Geometry: final body of the model. Coordinates: model frame, mm. Coordinates: 2 decimals unless noted, no trailing zeros. Write each loop counter-clockwise with the first axis right and the second up, starting at its lowest first coordinate (ties: lowest second). Pieces come first, ordered by that corner, then holes.
Autodesk Fusion 360 part; units mm, degrees
sketch "Esquisse1" plane through (0, 0, 0) normal (0, 0, 1) x (1, 0, 0)
  line L0 (74.9967, -34.0812) -> (-36.2033, -34.0812)
  circle A0 centre (59.0467, 6.2188) radius 15
  line L1 (76.9967, 28.1188) -> (76.9967, -32.0812)
  line L2 (-38.2033, -32.0812) -> (-38.2033, 28.1188)
  line L3 (74.8967, -31.9812) -> (-36.1033, -31.9812)
  line L4 (-36.2033, 30.1188) -> (74.9967, 30.1188)
  line L5 (-36.1033, 28.0188) -> (74.8967, 28.0188)
  line L6 (-36.1033, -31.9812) -> (-36.1033, 28.0188)
  circle A1 centre (8.0467, 6.2188) radius 15
  line L7 (74.8967, 28.0188) -> (74.8967, -31.9812)
  arc A2 (74.9967, -34.0812) -> (76.9967, -32.0812) centre (74.9967, -32.0812) ccw
  arc A3 (76.9967, 28.1188) -> (74.9967, 30.1188) centre (74.9967, 28.1188) ccw
  arc A4 (-36.2033, 30.1188) -> (-38.2033, 28.1188) centre (-36.2033, 28.1188) ccw
  arc A5 (-38.2033, -32.0812) -> (-36.2033, -34.0812) centre (-36.2033, -32.0812) ccw
  circle A6 centre (-19.1033, 10.5188) radius 6.5
  point P0 (-37.2797, 0.2421)
  dimension "d25" = 115.2
  dimension "d26" = 64.2
  dimension "d38" = 30
  dimension "d41" = 46.25
  dimension "d42" = 111
  dimension "d43" = 60
  dimension "d44" = 2.1
  dimension "d45" = 2.1
  dimension "d47" = 30
  dimension "d48" = 51
  dimension "d21" = 2
  dimension "d22" = 2
  dimension "d23" = 2
  dimension "d24" = 2
  dimension "d28" = 13
  dimension "d29" = 42.5
  dimension "d30" = 17
  dimension "d34" = 38.2
  dimension "d35" = 38.2
extrude "Extrusion1" add sketch "Esquisse1" along normal blind 1 contours L0 L1 L2 L4 A2 A3 A4 A5 | L3 L5 L6 L7
Item 1: Section B-B, the plane y = -2.5. Output: boundary loops of the cut face in (x, z), plus the area to 3 significant figures.
Derived:
outline: (-38.2, 0) - (-4.16, 0) - (-4.16, 1) - (-38.2, 1) - close; (20.25, 0) - (46.84, 0) - (46.84, 1) - (20.25, 1) - close; (71.25, 0) - (77, 0) - (77, 1) - (71.25, 1) - close
area: 66.4 mm2
Item 2: Pin query (flat end, axial travel): pin 1 (1.5 mm diameter, centred on x = 36, y = -22.5, fed in from -Z); pin 2 (8 mm diameter, centred on x = -19.1, y = 10.52, fed in from -Z). Return the tip coordinate at first contact, or that it passes through.
Derived:
pin 1: stops at z = 0
pin 2: passes through
Item 3: Section D-D, the plane x = 55. Output: boundary loops of the cut face in (y, z).
Derived:
outline: (-34.08, 0) - (-8.23, 0) - (-8.23, 1) - (-34.08, 1) - close; (20.66, 0) - (30.12, 0) - (30.12, 1) - (20.66, 1) - close
Item 4: Pull-direction query (Y, two-part tool) for faces 1 (the cylindrical face through (44.06, 5.56, 0.49)), 2 (the flat face through (19, -9, 0)), 3 (the cylindrical face through (-37.63, 29.52, 0.49)); classes: released by +Y, released by -Y, zero draft, split by the parting line, or undercut.
Derived:
face 1: undercut
face 2: zero draft
face 3: released by +Y
Item 5: Section C-C, the plane z = 0.4. Output: boundary loops of the cut face in (x, y).
Derived:
outline: (-38.2, -32.08) arc R2 ccw to (-36.2, -34.08) - (75, -34.08) arc R2 ccw to (77, -32.08) - (77, 28.12) arc R2 ccw to (75, 30.12) - (-36.2, 30.12) arc R2 ccw to (-38.2, 28.12) - close; hole circle Ø13 at (-19.1, 10.52); hole circle Ø30 at (8.05, 6.22); hole circle Ø30 at (59.05, 6.22)
Item 6: Material intervals for probe 1 along X at (y, z) = (-6, 0.1); probe 2 along X at (y, z) = (10, 0.8); probe 3 along X at (y, z) = (-4, 0.45), sorted ascending.
Derived:
probe 1: x = -38.2 to -0.65, 16.75 to 50.35, 67.75 to 77
probe 2: x = -38.2 to -25.58, -12.62 to -6.47, 22.56 to 44.53, 73.56 to 77
probe 3: x = -38.2 to -2.93, 19.03 to 48.07, 70.03 to 77
Item 7: Section A-A, the plane x = -22.5. Output: boundary loops of the cut face in (y, z), plus the area to 3 significant figures.
Derived:
outline: (-34.08, 0) - (4.98, 0) - (4.98, 1) - (-34.08, 1) - close; (16.06, 0) - (30.12, 0) - (30.12, 1) - (16.06, 1) - close
area: 53.1 mm2
